Check sheet for the modelled part. Datum: model origin and axes. Units: mm. Face numbers are marked on the shaded views. Coordinates: 2 decimals unless noted, no trailing zeros. Loops run counter-clockwise (first coordinate to the right, second up) from the corner with the lowest first, then second, coordinate; pieces in that order, holes last. Notation, with made-up numbers: (69.5, 86) -> (92.5, 86) arc R16 ccw to (92.5, 103) -> close; hole circle Ø8 at (34, 55). An arc over 180 degrees is marked (long way). Use one line per item in the form item = value.
from build123d import *

# Parameters (mm, degrees)
ESQUISSE1_W                     = 22
ESQUISSE1_H                     = 28
ESQUISSE1_R                     = 1.3
BOSS_EXTRU_1_DEPTH              = 1.7
ESQUISSE2_W                     = 6.33
ESQUISSE2_H                     = 5.17
BOSS_EXTRU_2_DEPTH              = 1.8
ESQUISSE3_R                     = 0.75
ENL_V_MAT_EXTRU_1_DEPTH         = 18.895250767
R_P_TITION_LIN_AIRE1_COUNT      = 8
R_P_TITION_LIN_AIRE1_PITCH      = 2.5
R_P_TITION_LIN_AIRE1_COUNT_DIR2 = 2
R_P_TITION_LIN_AIRE1_PITCH_DIR2 = 3
BOSS_EXTRU_3_START              = 0.25
ESQUISSE4_R                     = 1.267027295
ESQUISSE4_R_2                   = 0.75
BOSS_EXTRU_3_DEPTH              = 2.15
R_P_TITION_LIN_AIRE2_COUNT      = 8
R_P_TITION_LIN_AIRE2_PITCH      = 2.5
R_P_TITION_LIN_AIRE2_COUNT_DIR2 = 2
R_P_TITION_LIN_AIRE2_PITCH_DIR2 = 3


with BuildPart() as part:
    # Esquisse1 → Boss.-Extru.1 (new body)
    with BuildSketch(Plane.XY):
        Rectangle(ESQUISSE1_W, ESQUISSE1_H)
        with Locations((-9, -1)):
            Circle(ESQUISSE1_R, mode=Mode.SUBTRACT)
        with Locations((9, -1)):
            Circle(ESQUISSE1_R, mode=Mode.SUBTRACT)
        with Locations((9, -12)):
            Circle(ESQUISSE1_R, mode=Mode.SUBTRACT)
        with Locations((-9, -12)):
            Circle(ESQUISSE1_R, mode=Mode.SUBTRACT)
    extrude(amount=BOSS_EXTRU_1_DEPTH)

    # Esquisse2 → Boss.-Extru.2 (add)
    with BuildSketch(Plane.XY.offset(1.7)):
        with Locations((0, -6.5)):
            Rectangle(ESQUISSE2_W, ESQUISSE2_H)
    extrude(amount=BOSS_EXTRU_2_DEPTH)

    # Esquisse3 → Enlèv. mat.-Extru.1 (cut, through all)
    with BuildSketch(Plane.XY.offset(1.7)):
        with Locations((-8.47184488, 11.336604358)):
            Circle(ESQUISSE3_R)
    enl_v_mat_extru_1 = extrude(amount=-ENL_V_MAT_EXTRU_1_DEPTH, mode=Mode.SUBTRACT)

    # Répétition linéaire1: Enl_v. mat.-Extru.1 8 × 2
    with Locations(*[(i * R_P_TITION_LIN_AIRE1_PITCH, -j * R_P_TITION_LIN_AIRE1_PITCH_DIR2, 0) for i in range(R_P_TITION_LIN_AIRE1_COUNT) for j in range(R_P_TITION_LIN_AIRE1_COUNT_DIR2) if (i, j) != (0, 0)]):
        add(enl_v_mat_extru_1, mode=Mode.SUBTRACT)

    # Esquisse4 → Boss.-Extru.3 (add)
    with BuildSketch(Plane.XY.offset(1.7).offset(BOSS_EXTRU_3_START)):
        with Locations((-8.47184488, 11.336604358)):
            Circle(ESQUISSE4_R)
        with Locations((-8.47184488, 11.336604358)):
            Circle(ESQUISSE4_R_2, mode=Mode.SUBTRACT)
    boss_extru_3 = extrude(amount=-BOSS_EXTRU_3_DEPTH)

    # Répétition linéaire2: Boss.-Extru.3 8 × 2
    with Locations(*[(i * R_P_TITION_LIN_AIRE2_PITCH, -j * R_P_TITION_LIN_AIRE2_PITCH_DIR2, 0) for i in range(R_P_TITION_LIN_AIRE2_COUNT) for j in range(R_P_TITION_LIN_AIRE2_COUNT_DIR2) if (i, j) != (0, 0)]):
        add(boss_extru_3)


solid = part.part
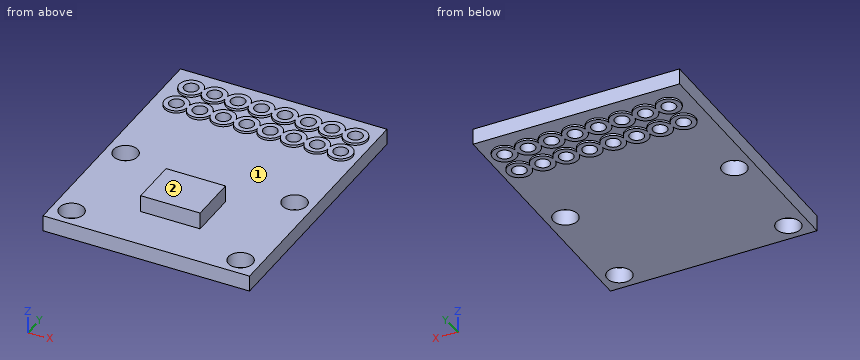
(1) Go/stop test with flat-tipped pins: P1, Ø2, axis at x = -3.47, y = 11.34, coming from the +Z side; P2, Ø4, axis at x = 9, y = -1, coming from the +Z side. Record where each tip stops, or that it passes through.
Established:
P1 = 1.95
P2 = 1.7
(2) Scan lines: line 1 along Y through (x, z) = (9, 0.55); line 2 along Y through (x, z) = (4, 0.3); line 3 along Y through (x, z) = (-1.5, 0.15). Record each from-to range of solid material in increasing order.
Established:
line_1 = -14 to -13.3, -10.7 to -2.3, 0.3 to 7.59, 9.09 to 10.59, 12.09 to 14
line_2 = -14 to 7.59, 9.09 to 10.59, 12.09 to 14
line_3 = -14 to 7.8, 8.87 to 10.8, 11.87 to 14
(3) Section check C-C, the plane y = -8.75. Record the boundary of the cut face in (x, z) (3 decimals).
Established:
outline = (-11, 0) -> (11, 0) -> (11, 1.7) -> (3.165, 1.7) -> (3.165, 3.5) -> (-3.165, 3.5) -> (-3.165, 1.7) -> (-11, 1.7) -> close
(4) Section check B-B, the plane y = -1. Record the boundary of the cut face in (x, z).
Established:
outline = (-11, 0) -> (-10.3, 0) -> (-10.3, 1.7) -> (-11, 1.7) -> close; (-7.7, 0) -> (7.7, 0) -> (7.7, 1.7) -> (-7.7, 1.7) -> close; (10.3, 0) -> (11, 0) -> (11, 1.7) -> (10.3, 1.7) -> close
(5) Mould release check, pull along Y, two halves, no side actions. Record for the marked faces 1 and 2: +Y half, -Y half, draft (parallel to the pull), parting line (faces both ways), or undercut.
Established:
face_1 = undercut
face_2 = draft
(6) Section check A-A, the plane x = 1.5. Give the number of separate pieces and of enclosed holes in the cut face, plus the area to 3 significant figures.
Established:
separate_pieces = 3
enclosed_holes = 0
area = 52.7 mm²
